```python
from build123d import *

# Parameters (mm, degrees)
EXTRUDE_1_DEPTH   = 4
EXTRUDE_1_2_DEPTH = 4
EXTRUDE_1_3_DEPTH = 4
SKETCH_2_W        = 7
SKETCH_2_H        = 5
EXTRUDE_2_DEPTH   = 0.6
SKETCH_3_W        = 4.85
SKETCH_3_H        = 1.2
EXTRUDE_3_DEPTH   = 0.6
SKETCH_4_W        = 1
SKETCH_4_H        = 13.65
EXTRUDE_4_DEPTH   = 0.6
FILLET_1_R        = 0.5
FILLET_2_R        = 0.3
SKETCH_5_W        = 1.1
SKETCH_5_H        = 0.6
EXTRUDE_5_DEPTH   = 2
FILLET_3_R        = 0.5


with BuildPart() as part:
    # Sketch 1 → Extrude 1 (new body)
    with BuildSketch(Plane(origin=(0, 0, 0), x_dir=(1, 0, 0), z_dir=(0, 1, 0))):
        with BuildLine():
            Line((-2.2, 1.245389122), (2.2, 1.245389122))
            ThreePointArc((2.2, 1.245389122), (2.694974747, 1.040363869), (2.9, 0.545389122))
            Line((2.9, 0.545389122), (2.9, -1.454610878))
            ThreePointArc((2.9, -1.454610878), (2.694974747, -1.949585625), (2.2, -2.154610878))
            Line((2.2, -2.154610878), (-2.2, -2.154610878))
            ThreePointArc((-2.2, -2.154610878), (-2.694974747, -1.949585625), (-2.9, -1.454610878))
            Line((-2.9, -1.454610878), (-2.9, 0.545389122))
            ThreePointArc((-2.9, 0.545389122), (-2.694974747, 1.040363869), (-2.2, 1.245389122))
        make_face()
    extrude(amount=EXTRUDE_1_DEPTH)



with BuildPart() as body_2:
    # Sketch 1 → Extrude 1 2 (new body)
    with BuildSketch(Plane(origin=(0, 0, 0), x_dir=(1, 0, 0), z_dir=(0, 1, 0))):
        with BuildLine():
            Line((-2.2, 7.528722779), (2.2, 7.528722779))
            ThreePointArc((2.2, 7.528722779), (2.694974747, 7.323697526), (2.9, 6.828722779))
            Line((2.9, 6.828722779), (2.9, 4.828722779))
            ThreePointArc((2.9, 4.828722779), (2.694974747, 4.333748032), (2.2, 4.128722779))
            Line((2.2, 4.128722779), (-2.2, 4.128722779))
            ThreePointArc((-2.2, 4.128722779), (-2.694974747, 4.333748032), (-2.9, 4.828722779))
            Line((-2.9, 4.828722779), (-2.9, 6.828722779))
            ThreePointArc((-2.9, 6.828722779), (-2.694974747, 7.323697526), (-2.2, 7.528722779))
        make_face()
    extrude(amount=EXTRUDE_1_2_DEPTH)


with BuildPart() as body_3:
    # Sketch 1 → Extrude 1 3 (new body)
    with BuildSketch(Plane(origin=(0, 0, 0), x_dir=(1, 0, 0), z_dir=(0, 1, 0))):
        with BuildLine():
            Line((-2.2, 13.775919566), (2.2, 13.775919566))
            ThreePointArc((2.2, 13.775919566), (2.694974747, 13.570894313), (2.9, 13.075919566))
            Line((2.9, 13.075919566), (2.9, 11.075919566))
            ThreePointArc((2.9, 11.075919566), (2.694974747, 10.580944819), (2.2, 10.375919566))
            Line((2.2, 10.375919566), (-2.2, 10.375919566))
            ThreePointArc((-2.2, 10.375919566), (-2.694974747, 10.580944819), (-2.9, 11.075919566))
            Line((-2.9, 11.075919566), (-2.9, 13.075919566))
            ThreePointArc((-2.9, 13.075919566), (-2.694974747, 13.570894313), (-2.2, 13.775919566))
        make_face()
    extrude(amount=EXTRUDE_1_3_DEPTH)


with BuildPart() as part_1:
    add(part.part)

    add(body_2.part)  # Extrude 2 merges body 2

    add(body_3.part)  # Extrude 2 merges body 3
    # Sketch 2 → Extrude 2 (add)
    with BuildSketch(Plane(origin=(0, 4, 0), x_dir=(1, 0, 0), z_dir=(0, 1, 0))):
        with Locations((0.036699987, 12.063062551)):
            Rectangle(SKETCH_2_W, SKETCH_2_H)
        with Locations((0.036699987, 5.863062551)):
            Rectangle(SKETCH_2_W, SKETCH_2_H)
        with Locations((0.036699987, -0.386937449)):
            Rectangle(SKETCH_2_W, SKETCH_2_H)
    extrude(amount=-EXTRUDE_2_DEPTH)

    # Sketch 3 → Extrude 3 (add)
    with BuildSketch(Plane(origin=(0, 4, 0), x_dir=(1, 0, 0), z_dir=(0, 1, 0))):
        with Locations((5.961699987, 12.063062551)):
            Rectangle(SKETCH_3_W, SKETCH_3_H)
        with Locations((5.961699987, 5.863062551)):
            Rectangle(SKETCH_3_W, SKETCH_3_H)
        with Locations((5.961699987, -0.386937449)):
            Rectangle(SKETCH_3_W, SKETCH_3_H)
    extrude(amount=-EXTRUDE_3_DEPTH)

    # Sketch 4 → Extrude 4 (add)
    with BuildSketch(Plane.XZ.offset(-3.4)):
        with Locations((7.886699987, -5.838062551)):
            Rectangle(SKETCH_4_W, SKETCH_4_H)
    extrude(amount=-EXTRUDE_4_DEPTH)

    # Fillet 1
    fillet_1_edges = [part_1.edges().sort_by_distance(p)[0] for p in [
        (3.536699987, 3.7, -11.463062551),
        (3.536699987, 3.7, -12.663062551),
        (3.536699987, 3.7, 0.986937449),
        (3.536699987, 3.7, -0.213062551),
        (3.536699987, 3.7, -5.263062551),
        (3.536699987, 3.7, -6.463062551),
    ]]
    fillet(fillet_1_edges, radius=FILLET_1_R)

    # Fillet 2
    fillet_2_edges = [part_1.edges().sort_by_distance(p)[0] for p in [
        (-2.9, 0, 0.454610878),
        (-2.694974747, 0, -1.040363869),
        (-2.694974747, 0, -13.570894313),
        (-2.9, 0, -12.075919566),
        (-2.694974747, 0, -10.580944819),
        (0, 0, -10.375919566),
        (2.694974747, 0, -10.580944819),
        (2.9, 0, -12.075919566),
        (2.694974747, 0, -13.570894313),
        (0, 0, -13.775919566),
        (0, 0, -1.245389122),
        (2.694974747, 0, -1.040363869),
        (2.9, 0, 0.454610878),
        (2.694974747, 0, 1.949585625),
        (-2.694974747, 0, -7.323697526),
        (-2.9, 0, -5.828722779),
        (-2.694974747, 0, -4.333748032),
        (0, 0, -4.128722779),
        (2.694974747, 0, -4.333748032),
        (2.9, 0, -5.828722779),
        (0, 0, 2.154610878),
        (2.694974747, 0, -7.323697526),
        (0, 0, -7.528722779),
        (-2.694974747, 0, 1.949585625),
    ]]
    fillet(fillet_2_edges, radius=FILLET_2_R)

    # Sketch 5 → Extrude 5 (add)
    with BuildSketch(Plane(origin=(0, 0, -12.663062551), x_dir=(-1, 0, 0), z_dir=(0, 0, -1))):
        with Locations((-7.836699987, 3.7)):
            Rectangle(SKETCH_5_W, SKETCH_5_H)
    extrude(amount=EXTRUDE_5_DEPTH)

    # Fillet 3
    fillet_3_edges = [part_1.edges().sort_by_distance(p)[0] for p in [
        (7.836699987, 3.4, -14.663062551),
    ]]
    fillet(fillet_3_edges, radius=FILLET_3_R)


solid = part_1.part
```
Check sheet for the modelled part. Datum: model origin and axes. Units: mm. A direction names the side the tool comes from. Coordinates: 2 decimals unless noted, no trailing zeros. Order: outer loops, then holes, each group sorted by start corner. A loop starts at its lowest first (then second) coordinate and runs counter-clockwise, first axis right, second up. Notation, with made-up numbers: M -32,13.25 L 26,13.25 A16 cw 26,41.25 Z; hole C 3.25,27 d1. An arc over 180 degrees is marked long. One line per question, with ' | ' between items. Start each with the question number.
Item 1: Sectioned sample at A-A on x = -1.25. Count the separate pieces of the cut face and the enclosed holes in it, and give its area (3 significant figures).
Item 2: Gauge pin test, flat ends, axial feed: P1, Ø1, axis at x = -2.5, y = 1.5, coming from the +Z side; P2, Ø0.9, axis at x = -0.5, y = 1.5, coming from the -Z side; P3, Ø0.7, axis at x = 6, y = 4, coming from the +Z side. Record the tip position at first contact, or that the pin passes through.
Item 3: Access from +Z, -Z, +X, -X, +Y, -Y to the whole of each face (thin tool, end or side, straight path). Record for faces 4 (the flat face through (0, 2, -13.776)), 5 (the flat face through (-2.9, 2, -12)), 6 (the flat face through (0, 2, -1.245)), 7 (the flat face through (2.9, 2, -12)).
Item 4: Sectioned sample at C-C on z = -11.25. Record the cut outline in (x, y).
Item 5: Sectioned sample at B-B on y = 2.95. Record the cut outline in (x, z).
Item 6: Material ranges on line 1 (Z direction, x = -1.75, y = 2.35); line 2 (Z direction, x = 3, y = 3.7); line 3 (X direction, y = 1.9, z = -5.5), recorded low to high.
Item 7: Sectioned sample at D-D on x = 6.5. Record the cut outline in (y, z), and give its area (3 significant figures).
Item 8: Mould release check, pull along Z, two halves, no side actions. Record for faces 1 (the flat face through (-2.9, 2, -6)), 2 (the flat face through (0, 2, -7.529)), 3 (the flat face through (0, 2, 2.155)): pulls with the +Z half, pulls with the -Z half, needs draft (parallel to the pull), parting line crosses it, or undercut.
Answer below:
1) separate pieces: 3 | enclosed holes: 0 | area: 43.6 mm^2
2) P1: stops at z = 2.15 | P2: stops at z = -13.78 | P3: stops at z = 0.99
3) face 4: -Z, +X, -X, -Y | face 5: +Z, -Z, -X, -Y | face 6: +X, -X, -Y | face 7: +Z, -Z, +X, -Y
4) outline: M -3.46,3.4 L -2.9,3.4 L -2.9,0.3 A0.3 ccw -2.6,0 L 2.6,0 A0.3 ccw 2.9,0.3 L 2.9,3.4 L 3.63,3.4 L 3.63,4 L -3.46,4 Z; M 7.39,3.4 L 8.39,3.4 L 8.39,4 L 7.39,4 Z
5) outline: M -2.9,-13.08 A0.7 ccw -2.2,-13.78 L 2.2,-13.78 A0.7 ccw 2.9,-13.08 L 2.9,-11.08 A0.7 ccw 2.2,-10.38 L -2.2,-10.38 A0.7 ccw -2.9,-11.08 Z; M -2.9,-6.83 A0.7 ccw -2.2,-7.53 L 2.2,-7.53 A0.7 ccw 2.9,-6.83 L 2.9,-4.83 A0.7 ccw 2.2,-4.13 L -2.2,-4.13 A0.7 ccw -2.9,-4.83 Z; M -2.9,-0.55 A0.7 ccw -2.2,-1.25 L 2.2,-1.25 A0.7 ccw 2.9,-0.55 L 2.9,1.45 A0.7 ccw 2.2,2.15 L -2.2,2.15 A0.7 ccw -2.9,1.45 Z
6) line 1: z = -13.78 to -10.38, -7.53 to -4.13, -1.25 to 2.15 | line 2: z = -14.56 to -9.56, -8.36 to -3.36, -2.11 to 2.89 | line 3: x = -2.9 to 2.9
7) outline: M 3.4,-12.66 L 4,-12.66 L 4,-11.46 L 3.4,-11.46 Z; M 3.4,-6.46 L 4,-6.46 L 4,-5.26 L 3.4,-5.26 Z; M 3.4,-0.21 L 4,-0.21 L 4,0.99 L 3.4,0.99 Z | area: 2.16 mm^2
8) face 1: needs draft | face 2: undercut | face 3: pulls with the +Z half
